Input: part model. Units: mm. Frame: model coordinates. A direction names the side the tool comes from. Give positions to 0.01 mm unless a question says otherwise; leave off trailing zeros. Loops run counter-clockwise (first coordinate to the right, second up) from the corner with the lowest first, then second, coordinate; pieces in that order, holes last. Notation, with made-up numbers: (49, 12) -> (97, 12) arc R22 ccw to (97, 44) -> close; hole circle Ø9 at (5, 27). An arc over 180 degrees is marked (long way). Answer as a JSON object with one key per item and string values.
```python
from build123d import *

# Parameters (mm, degrees)
SKETCH2_OUTSIDE_W  = 29.014
SKETCH2_OUTSIDE_H  = 29.014
CUT_EXTRUDE1_DEPTH = 56.367668431
CHAMFER1_SIZE      = 0.508


with BuildPart() as part:
    # Sketch1 → Revolve1 (revolve)
    with BuildSketch(Plane(origin=(0, 0, 0), x_dir=(0, 0, -1), z_dir=(1, 0, 0)), mode=Mode.PRIVATE) as revolve1_sk:
        Polygon((0, 2.5527), (0, 6.35), (7.9502, 6.35), (7.9502, 5.842), (8.9408, 5.842), (8.9408, 6.8707), (19.88570353, 6.8707), (54.5084, 6.8707), (54.5084, 5.842), (55.499, 5.842), (55.499, 6.35), (63.4492, 6.35), (63.4492, 2.5527), (19.88570353, 2.5527), align=None)
    revolve(revolve1_sk.sketch.rotate(Axis((0, 0, 0), (0, 0, 1)), 90), axis=Axis((0, 0, 0), (0, 0, 1)))

    # Sketch2 outside → Cut-Extrude1 (cut, through all)
    with BuildSketch(Plane.XY.offset(-8.9408)):
        Rectangle(SKETCH2_OUTSIDE_W, SKETCH2_OUTSIDE_H)
        Polygon((-3.666174209, 6.35), (-7.332348419, 0), (-3.666174209, -6.35), (3.666174209, -6.35), (7.332348419, 0), (3.666174209, 6.35), align=None, mode=Mode.SUBTRACT)
    extrude(amount=-CUT_EXTRUDE1_DEPTH, mode=Mode.SUBTRACT)

    # Chamfer1
    chamfer1_edges = [part.edges().sort_by_distance(p)[0] for p in [
        (6.35, 0, -63.4492),
        (6.35, 0, 0),
    ]]
    chamfer(chamfer1_edges, length=CHAMFER1_SIZE)


solid = part.part
```
Q1. Access query for faces 1 (the cylindrical face through (5.04, 3.86, -59.27)), 2 (the flat face through (-2, -6, -8.941)), 3 (the cylindrical face through (5.04, 3.86, -4.28)). Directions: +Z, -Z, +X, -X, +Y, -Y. A direction counts if a zero-diameter tool reaches every point of the face in a straight line with its end or side. Return the directions, or none.
Evaluation:
{"face 1": "-Z", "face 2": "none", "face 3": "+Z"}
Q2. Section A-A, the plane x = 0. Return the cut outline in (y, z), then the cut area to 3 significant figures.
Evaluation:
{"outline": "(-6.35, -62.94) -> (-5.84, -63.45) -> (-2.55, -63.45) -> (-2.55, 0) -> (-5.84, 0) -> (-6.35, -0.51) -> (-6.35, -7.95) -> (-5.84, -7.95) -> (-5.84, -8.94) -> (-6.35, -8.94) -> (-6.35, -54.51) -> (-5.84, -54.51) -> (-5.84, -55.5) -> (-6.35, -55.5) -> close; (2.55, -63.45) -> (5.84, -63.45) -> (6.35, -62.94) -> (6.35, -55.5) -> (5.84, -55.5) -> (5.84, -54.51) -> (6.35, -54.51) -> (6.35, -8.94) -> (5.84, -8.94) -> (5.84, -7.95) -> (6.35, -7.95) -> (6.35, -0.51) -> (5.84, 0) -> (2.55, 0) -> close", "area": "479 mm2"}
Q3. Ray query, line 1 along Y through (x, z) = (0, -53); line 2 along X through (y, z) = (-0.25, -31); line 3 along Z through (x, y) = (-6, -0.25). Return the intervals inside material, ascending.
Evaluation:
{"line 1": "y = -6.35 to -2.55, 2.55 to 6.35", "line 2": "x = -6.87 to -2.54, 2.54 to 6.87", "line 3": "z = -63.29 to -55.5, -54.51 to -8.94, -7.95 to -0.16"}
Q4. Section B-B, the plane z = -23. Return the cut outline in (x, y), then the cut area to 3 significant figures.
Evaluation:
{"outline": "(-6.81, -0.9) -> (-4.19, -5.45) arc R6.87 ccw to (-2.62, -6.35) -> (2.62, -6.35) arc R6.87 ccw to (4.19, -5.45) -> (6.81, -0.9) arc R6.87 ccw to (6.81, 0.9) -> (4.19, 5.45) arc R6.87 ccw to (2.62, 6.35) -> (-2.62, 6.35) arc R6.87 ccw to (-4.19, 5.45) -> (-6.81, 0.9) arc R6.87 ccw to start; hole circle Ø5.11 at (0, 0)", "area": "117 mm2"}
Q5. Draft query along Y for faces 4 (the flat face through (-1, 3, -63.449)), 5 (the cylindrical face through (6.87, -0.01, -31.41)), 6 (the cylindrical face through (-2.435, -0.767, -32.169)). Return one class per face: +Y half, -Y half, draft (parallel to the pull), parting line (faces both ways), or undercut.
Evaluation:
{"face 4": "draft", "face 5": "parting line", "face 6": "undercut"}
Q6. Pin query (flat end, axial travel): pin 1 (5 mm diameter, centred on x = -0.5, y = -2.5, fed in from +Z); pin 2 (1 mm diameter, centred on y = -1, z = -18.5, fed in from -X); pin 3 (1 mm diameter, centred on y = 3, z = -54, fed in from +X); pin 4 (1 mm diameter, centred on x = 4, z = -33, fed in from +Y). Return the tip coordinate at first contact, or that it passes through.
Evaluation:
{"pin 1": "stops at z = 0", "pin 2": "stops at x = -6.85", "pin 3": "stops at x = 5.89", "pin 4": "stops at y = 5.91"}
Q7. Section C-C, the plane y = 0. Return the cut outline in (x, z), then the cut area to 3 significant figures.
Evaluation:
{"outline": "(-6.87, -54.51) -> (-5.84, -54.51) -> (-5.84, -55.5) -> (-6.35, -55.5) -> (-6.35, -62.94) -> (-5.84, -63.45) -> (-2.55, -63.45) -> (-2.55, 0) -> (-5.84, 0) -> (-6.35, -0.51) -> (-6.35, -7.95) -> (-5.84, -7.95) -> (-5.84, -8.94) -> (-6.87, -8.94) -> close; (2.55, -63.45) -> (5.84, -63.45) -> (6.35, -62.94) -> (6.35, -55.5) -> (5.84, -55.5) -> (5.84, -54.51) -> (6.87, -54.51) -> (6.87, -8.94) -> (5.84, -8.94) -> (5.84, -7.95) -> (6.35, -7.95) -> (6.35, -0.51) -> (5.84, 0) -> (2.55, 0) -> close", "area": "527 mm2"}
